from build123d import *

# Parameters (mm, degrees)
BOSS_EXTRUDE1_DEPTH = 45
CUT_EXTRUDE1_DEPTH  = 2
SKETCH4_W           = 10
SKETCH4_H           = 2
CUT_EXTRUDE2_DEPTH  = 2
SKETCH5_W           = 20
SKETCH5_H           = 2
BOSS_EXTRUDE2_DEPTH = 10
SKETCH6_R           = 1.5
CUT_EXTRUDE3_DEPTH  = 2


with BuildPart() as part:
    # Sketch1 → Boss-Extrude1 (new body)
    with BuildSketch(Plane.XY):
        Polygon((0, 0), (6, 0), (6, 20), (8, 20), (8, -2), (-2, -2), (-2, 20), (0, 20), align=None)
    extrude(amount=BOSS_EXTRUDE1_DEPTH)

    # Sketch3 → Cut-Extrude1 (cut)
    with BuildSketch(Plane.ZY.offset(2)):
        with BuildLine():
            ThreePointArc((43.6, 9.407510361), (35.6, 17.407510361), (27.6, 9.407510361))
            Line((27.6, 9.407510361), (43.6, 9.407510361))
        make_face()
        with BuildLine():
            Line((43.6, 9.407510361), (27.6, 9.407510361))
            ThreePointArc((27.6, 9.407510361), (35.6, 1.407510361), (43.6, 9.407510361))
        make_face()
        with BuildLine():
            Line((1.4, 20), (1.4, 9.407510361))
            ThreePointArc((1.4, 9.407510361), (9.4, 17.407510361), (17.4, 9.407510361))
            Line((17.4, 9.407510361), (17.4, 20))
            Line((17.4, 20), (1.4, 20))
        make_face()
        with BuildLine():
            ThreePointArc((17.4, 9.407510361), (9.4, 17.407510361), (1.4, 9.407510361))
            Line((1.4, 9.407510361), (17.4, 9.407510361))
        make_face()
        with BuildLine():
            Line((17.4, 9.407510361), (1.4, 9.407510361))
            ThreePointArc((1.4, 9.407510361), (9.4, 1.407510361), (17.4, 9.407510361))
        make_face()
        with BuildLine():
            Line((43.6, 20), (27.6, 20))
            Line((27.6, 20), (27.6, 9.407510361))
            ThreePointArc((27.6, 9.407510361), (35.6, 17.407510361), (43.6, 9.407510361))
            Line((43.6, 9.407510361), (43.6, 20))
        make_face()
    extrude(amount=-CUT_EXTRUDE1_DEPTH, mode=Mode.SUBTRACT)

    # Sketch4 → Cut-Extrude2 (cut)
    with BuildSketch(Plane(origin=(8, 0, 0), x_dir=(0, 0, -1), z_dir=(1, 0, 0))):
        with Locations((-22.5, 19)):
            Rectangle(SKETCH4_W, SKETCH4_H)
    extrude(amount=-CUT_EXTRUDE2_DEPTH, mode=Mode.SUBTRACT)

    # Sketch5 → Boss-Extrude2 (add)
    with BuildSketch(Plane(origin=(8, 0, 0), x_dir=(0, 0, -1), z_dir=(1, 0, 0))):
        with Locations((-22.5, -1)):
            Rectangle(SKETCH5_W, SKETCH5_H)
    extrude(amount=BOSS_EXTRUDE2_DEPTH)

    # Sketch6 → Cut-Extrude3 (cut)
    with BuildSketch(Plane(origin=(0, 0, 0), x_dir=(1, 0, 0), z_dir=(0, 1, 0))):
        with Locations(Location((12.760241106, -27.5, 0), (0, 0, 180))):
            Circle(SKETCH6_R)
        with Locations(Location((12.760241106, -17.5, 0), (0, 0, 180))):
            Circle(SKETCH6_R)
    extrude(amount=-CUT_EXTRUDE3_DEPTH, mode=Mode.SUBTRACT)


solid = part.part
The listing builds one solid part. Answer for the finished solid, in the listing's coordinates (mm). A direction names the side the tool comes from. Round coordinates to 2 decimals unless told otherwise and drop trailing zeros. Write each loop counter-clockwise with the first axis right and the second up, starting at its lowest first coordinate (ties: lowest second). Pieces come first, ordered by that corner, then holes. Notation, with made-up numbers: M 12.5,71.25 L 70.5,71.25 A23 ccw 70.5,86.25 Z; hole C 64.5,81.25 d7. An arc over 180 degrees is marked long. Write each question's results on one line, items separated by ' | '. Start each with the question number.
Item 1: Straight lines are drawn through the part: L1, parallel to Y at x = 9.5, z = 29; L2, parallel to X at y = 3, z = 8.5. For each, find the intervals that lie inside material, in ascending order. Write a range as [from, to].
Item 2: For faces 1 (the face through (13, -1, 32.5)), 2 (the face through (13, -1, 12.5)), 3 (the face through (6, 10, 22)), determine the directions among +Z, -Z, +X, -X, +Y, -Y from which every point of the face is accessible in a straight line to the end or side of a thin tool.
Item 3: A cutting plane is placed at B-B on y = 0.5. Write down the section's boundary in (x, z).
Item 4: For a pull along X with two mould halves and no side action, classify faces 4 (the face through (13, 0, 23)), 5 (the face through (0, 8, 22)), 6 (the face through (18, -1, 23)) as pulls with the +X half, pulls with the -X half, needs draft (parallel to the pull), parting line crosses it, or undercut.
Item 5: A cutting plane is placed at C-C on z = 35.6. Write down the section's boundary in (x, y).
Item 6: A cutting plane is placed at A-A on y = 17.25. Write down the section's boundary in (x, z), and give its area (3 significant figures).
Item 7: Flat-ended cylindrical pins translate along their axes: pin 1 Ø1.6 at (x, y) = (11.5, -1.5) entering from +Z; pin 2 Ø5 at (x, z) = (11, 26) entering from +Y; pin 3 Ø6.5 at (x, z) = (2, 30) entering from +Y; pin 4 Ø2 at (x, z) = (6.5, 23) entering from +Y. Find the tip coordinate at first contact, or state that the pin passes through.
Item 8: A cutting plane is placed at D-D on z = 18. Write down the section's boundary in (x, y), and give its area (3 significant figures).
Check sheet entries:
1) L1: [-2, 0] | L2: [6, 8]
2) face 1: +Z, +X, +Y, -Y | face 2: -Z, +X, +Y, -Y | face 3: +Z, -Z, +Y
3) outline: M -2,0 L 0,0 L 0,45 L -2,45 Z; M 6,0 L 8,0 L 8,45 L 6,45 Z
4) face 4: needs draft | face 5: undercut | face 6: pulls with the +X half
5) outline: M -2,-2 L 8,-2 L 8,20 L 6,20 L 6,0 L 0,0 L 0,1.41 L -2,1.41 Z
6) outline: M -2,0 L 0,0 L 0,1.4 L -2,1.4 Z; M -2,17.4 L 0,17.4 L 0,27.6 L -2,27.6 Z; M -2,43.6 L 0,43.6 L 0,45 L -2,45 Z; M 6,0 L 8,0 L 8,45 L 6,45 Z | area: 116 mm²
7) pin 1: z = 32.5 | pin 2: y = 0 | pin 3: y = 20 | pin 4: y = 18
8) outline: M -2,-2 L 11.35,-2 L 11.35,0 L 8,0 L 8,18 L 6,18 L 6,0 L 0,0 L 0,20 L -2,20 Z; M 14.17,-2 L 18,-2 L 18,0 L 14.17,0 Z | area: 110 mm²
